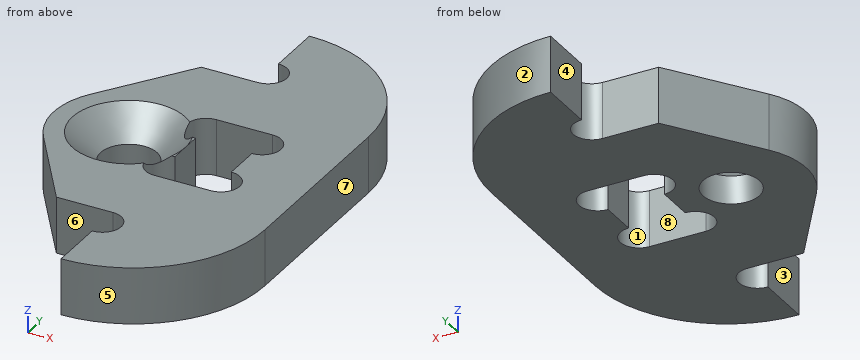
Autodesk Inventor part; units mm, degrees
ref_plane "YZ Plane" through (0, 0, 0) normal (1, 0, 0) x (0, 1, 0)
ref_plane "XZ Plane" through (0, 0, 0) normal (0, 1, 0) x (-1, 0, 0)
ref_plane "XY Plane" through (0, 0, 0) normal (0, 0, 1) x (1, 0, 0)
sketch "スケッチ5" plane through (0, 0, 0) normal (0, 0, 1) x (1, 0, 0)
  line L0 (-1, 1) -> (-1, -1)
  circle A0 centre (-4, 0) radius 1.5
  arc A1 (2, 1) -> (2, 3) centre (2, 2) ccw
  arc A2 (2, -3) -> (2, -1) centre (2, -2) ccw
  arc A3 (-1, 3) -> (-1, 1) centre (-1, 2) ccw
  arc A4 (-1, -1) -> (-1, -3) centre (-1, -2) ccw
  line L1 (2, -3) -> (-1, -3)
  line L2 (-1, 3) -> (2, 3)
  arc A5 (-7.2826, 2.2857) -> (-7.2826, -2.2857) centre (-4, 0) ccw
  line L3 (-1, -7) -> (-1, -7)
  line L4 (6, -5) -> (6, 5)
  line L5 (-1, 7) -> (-1, 7)
  line L6 (0, 0) -> (-1, 0) construction
  arc A6 (-1, -9) -> (-1, -7) centre (-1, -8) ccw
  line L7 (-1, -9) -> (-1, -12)
  arc A7 (-1, -12) -> (6, -5) centre (-1, -5) ccw
  arc A8 (6, 5) -> (-1, 12) centre (-1, 5) ccw
  line L8 (-1, 12) -> (-1, 9)
  arc A9 (-1, 7) -> (-1, 9) centre (-1, 8) ccw
  line L9 (2, -1) -> (2, 1)
  line L10 (-7.2826, -2.2857) -> (-4, -7)
  line L11 (-4, -7) -> (-1, -7)
  line L12 (-7.2826, 2.2857) -> (-4, 7)
  line L13 (-4, 7) -> (-1, 7)
  point P0 (2, 0)
  point P1 (6, 0)
  point P2 (2, 0)
  dimension "d57" = 3
  dimension "d58" = 2
  dimension "d60" = 4
  dimension "d61" = 4
  dimension "d62" = 3
  dimension "d63" = 14
  dimension "d65" = 4
  dimension "d66" = 3
  dimension "d67" = 2
  dimension "d68" = 3
  dimension "d69" = 6
  dimension "d72" = 3
extrude "押し出し2" add sketch "スケッチ5" along normal blind 3
chamfer "面取り2" distance 1.5 angle 45 1 edges at (-5.5, 0, 3)
properties part number "ShaftBase2"
CAD build for the part. Positions are in the model's coordinates, mm. Face numbers are marked on the shaded views. A direction names the side the tool comes from. Round coordinates to 2 decimals unless told otherwise and drop trailing zeros. Loops run counter-clockwise (first coordinate to the right, second up) from the corner with the lowest first, then second, coordinate; pieces in that order, holes last.
(1) Cut at C-C (y = 10.5). Give the cut face in (x, z), plus the area to 3 significant figures.
(2) Cut at A-A (z = 2.05). Give the cut face in (x, y), plus the area to 3 significant figures.
(3) Cut at B-B (y = -8). Give the cut face in (x, z).
(4) Which spindle directions (+Z, -Z, +X, -X, +Y, -Y) get a long thin tool onto all of the face, cutting with end or side? Do the marked faces 1, 2, 3, 4 and 5. Say none if no direction does.
(5) Drop flat-ended pins along their axis: pin 1 (4 mm diameter, centred on x = -4, y = 0, fed in from +Z); pin 2 (1 mm diameter, centred on y = 8.5, z = 0.5, fed in from +X); pin 3 (1.5 mm diameter, centred on y = 10, z = 1.5, fed in from -X). Give the stop position or say it passes through.
(6) Wall check: line 1 along X through (y, z) = (0, 2.45); line 2 along Y through (x, z) = (-3.5, 0.85); line 3 along Y through (x, z) = (-5, 1.2). Give the ranges that are in metal, low to high.
(7) Two-plate mould, pull along X, no slides. Class the marked faces 6, 7 and 8: +X half, -X half, draft (parallel to the pull), parting line (faces both ways), or undercut.
Findings below:
1. outline: (-1, 0) - (3.33, 0) - (3.33, 3) - (-1, 3) - close
1. area: 13.0 mm2
2. outline: (-7.28, -2.29) - (-4, -7) - (-1, -7) arc R1 cw to (-1, -9) - (-1, -12) arc R7 ccw to (6, -5) - (6, 5) arc R7 ccw to (-1, 12) - (-1, 9) arc R1 cw to (-1, 7) - (-4, 7) - (-7.28, 2.29) arc R4 ccw to start; hole circle Ø4.1 at (-4, 0); hole (-1, -3) - (2, -3) arc R1 ccw to (2, -1) - (2, 1) arc R1 ccw to (2, 3) - (-1, 3) arc R1 ccw to (-1, 1) - (-1, -1) arc R1 ccw to start
2. area: 181 mm2
3. outline: (0, 0) - (5.32, 0) - (5.32, 3) - (0, 3) - close
4. face 1: +Z, -Z
4. face 2: +Z, -Z, +X, +Y
4. face 3: +Z, -Z, -X, -Y
4. face 4: +Z, -Z, -X, +Y
4. face 5: +Z, -Z, +X, -Y
5. pin 1: stops at z = 2
5. pin 2: stops at x = 5.32
5. pin 3: stops at x = -1
6. line 1: x = -8 to -6.45, -1.55 to -1, 2 to 6
6. line 2: y = -7 to -1.41, 1.41 to 7
6. line 3: y = -5.56 to -1.12, 1.12 to 5.56
7. face 6: draft
7. face 7: +X half
7. face 8: undercut
